Input: part model. Units: mm. Frame: model coordinates. A direction names the side the tool comes from. Give positions to 0.01 mm unless a question says otherwise; leave off trailing zeros. Loops run counter-clockwise (first coordinate to the right, second up) from the corner with the lowest first, then second, coordinate; pieces in that order, holes last. Notation, with made-up numbers: (-23.75, 28.5) -> (17.25, 28.5) arc R21 ccw to (17.25, 64.5) -> close; hole circle Ø3 at (-32.5, -5.75). An arc over 180 degrees is marked (long way). One line per question, with ' | ' between items.
from build123d import *

# Parameters (mm, degrees)
SKETCH1_R           = 5
SKETCH1_R_2         = 2.5
BOSS_EXTRUDE1_DEPTH = 5
CUT_EXTRUDE2_DEPTH  = 5
FILLET1_R           = 5
CUT_EXTRUDE3_DEPTH  = 69.190908485
FILLET2_R           = 5


with BuildPart() as part:
    # Sketch1 → Boss-Extrude1 (new body)
    # profile 1 of 4: a face of its own
    with BuildSketch(Plane.XY):
        with BuildLine():
            Line((5, -15), (5, 60))
            ThreePointArc((5, 60), (-0.663665755, 55.04424095), (-4.823819106, 61.315587029))
            Line((-4.823819106, 61.315587029), (-19.823819106, 6.315587029))
            ThreePointArc((-19.823819106, 6.315587029), (-14.336334245, 9.95575905), (-10, 5))
            ThreePointArc((-10, 5), (-13.41886117, 0.25658351), (-19, 2))
            Line((-19, 2), (-4, -18))
            ThreePointArc((-4, -18), (-1.58113883, -10.25658351), (5, -15))
        make_face()
    # profile 2 of 4: a face of its own
    with BuildSketch(Plane.XY):
        with Locations((-15, 5)):
            Circle(SKETCH1_R)
        with Locations((-15, 5)):
            Circle(SKETCH1_R_2, mode=Mode.SUBTRACT)
    # profile 3 of 4: a face of its own
    with BuildSketch(Plane.XY):
        with Locations((0, -15)):
            Circle(SKETCH1_R)
        with Locations((0, -15)):
            Circle(SKETCH1_R_2, mode=Mode.SUBTRACT)
    # profile 4 of 4: a face of its own
    with BuildSketch(Plane.XY):
        with Locations((0, 60)):
            Circle(SKETCH1_R)
        with Locations((0, 60)):
            Circle(SKETCH1_R_2, mode=Mode.SUBTRACT)
    extrude(amount=BOSS_EXTRUDE1_DEPTH)

    # Sketch3 → Cut-Extrude2 (cut)
    with BuildSketch(Plane.XY.offset(5)):
        Polygon((5, 12.990381057), (5, -4.330127019), (-2.5, 0), align=None)
    extrude(amount=-CUT_EXTRUDE2_DEPTH, mode=Mode.SUBTRACT)

    # Fillet1
    fillet1_edges = [part.edges().sort_by_distance(p)[0] for p in [
        (-2.5, 0, 2.5),
        (5, 12.990381057, 2.5),
        (5, -4.330127019, 2.5),
    ]]
    fillet(fillet1_edges, radius=FILLET1_R)

    # Sketch4 → Cut-Extrude3 (cut, through all)
    with BuildSketch(Plane.XY.offset(5)):
        with BuildLine():
            Line((-9.110982773, 45.595986917), (-16.418905931, 18.800268672))
            ThreePointArc((-16.418905931, 18.800268672), (-6.155108901, 30.395445399), (-9.110982773, 45.595986917))
        make_face()
    extrude(amount=-CUT_EXTRUDE3_DEPTH, mode=Mode.SUBTRACT)

    # Fillet2
    fillet2_edges = [part.edges().sort_by_distance(p)[0] for p in [
        (-9.110982773, 45.595986917, 2.5),
        (-16.418905931, 18.800268672, 2.5),
    ]]
    fillet(fillet2_edges, radius=FILLET2_R)


solid = part.part
1. Section query C-C (y = 24). Output: boundary loops of the cut face in (x, z).
Determined:
outline: (-9.43, 0) -> (5, 0) -> (5, 5) -> (-9.43, 5) -> close
2. Pin query (flat end, axial travel): P1, Ø2, axis at x = -3.5, z = 4.5, coming from the -Y side; P2, Ø1, axis at y = 42, z = 2, coming from the -X side; P3, Ø1, axis at y = -9.5, z = 4, coming from the -X side; P4, Ø1, axis at x = -8.5, y = 48, coming from the -Z side. Return the tip coordinate at first contact, or that it passes through.
Determined:
P1: stops at y = -19.33 | P2: stops at x = -7.23 | P3: stops at x = -10.75 | P4: stops at z = 0
3. Section query D-D (y = 36.5). Output: boundary loops of the cut face in (x, z), then the cut area to 3 significant figures.
Determined:
outline: (-5.6, 0) -> (5, 0) -> (5, 5) -> (-5.6, 5) -> close | area: 53.0 mm2
4. Reachability of faces 4 (the flat face through (-18.4, 11.53, 2.46)), 5 (the flat face through (2.135, 8.028, 2.535)) from +Z, -Z, +X, -X, +Y, -Y: full face, straight path, thin tool, end or side. Return the list, or none.
Determined:
face 4: +Z, -Z, -X, +Y | face 5: +Z, -Z, +X
5. Ray query, line 1 along Y through (x, z) = (0, 1); line 2 along X through (y, z) = (59, 0.55); line 3 along X through (y, z) = (60.5, 3.2). Return the intervals inside material, ascending. Write a range as from..to.
Determined:
line 1: y = -20..-17.5, -12.5..-0.67, 4.33..57.5, 62.5..65 | line 2: x = -5.46..-2.29, 2.29..5 | line 3: x = -5.05..-2.45, 2.45..4.97
6. Pull-direction query (X, two-part tool) for faces 1 (the cylindrical face through (-0.54, -17.44, 2.46)), 2 (the cylindrical face through (4.834, 13.054, 2.465)), 3 (the flat face through (-11.605, -7.86, 2.465)); classes: pulls with the +X half, pulls with the -X half, needs draft (parallel to the pull), parting line crosses it, or undercut.
Determined:
face 1: undercut | face 2: pulls with the +X half | face 3: pulls with the -X half
7. Section query B-B (x = -13.75). Output: boundary loops of the cut face in (y, z).
Determined:
outline: (-5, 0) -> (2.83, 0) -> (2.83, 5) -> (-5, 5) -> close; (7.17, 0) -> (20.17, 0) -> (20.17, 5) -> (7.17, 5) -> close
8. Section query A-A (z = 2.5). Output: boundary loops of the cut face in (x, y).
Determined:
outline: (-19.82, 6.32) arc R5 ccw to (-19, 2) -> (-4, -18) arc R5 ccw to (5, -15) -> (5, -7.22) arc R5 ccw to (2.5, -2.89) -> (1.83, -2.5) arc R5 cw to (0, 4.33) -> (4.33, 11.83) arc R5 ccw to (5, 14.33) -> (5, 60) arc R5 ccw to (-4.82, 61.32) -> (-8.51, 47.8) arc R5 ccw to (-7.99, 43.93) arc R17.5 cw to (-14.6, 19.67) arc R5 ccw to (-17.02, 16.6) -> close; hole circle Ø5 at (-15, 5); hole circle Ø5 at (0, -15); hole circle Ø5 at (0, 60)
